```python
from build123d import *

# Parameters (mm, degrees)
BOSS_EXTRUDE1_DEPTH = 17.78
SKETCH4_R           = 1.905
SKETCH4_R_2         = 1.1
SKETCH4_W           = 3.81
SKETCH4_H           = 6.35
CUT_EXTRUDE1_DEPTH  = 7.62
BOSS_EXTRUDE2_DEPTH = 1.27
BOSS_EXTRUDE3_DEPTH = 1.27
FILLET1_R           = 3.81


with BuildPart() as part:
    # Sketch3 → Boss-Extrude1 (new body)
    with BuildSketch(Plane(origin=(0, 0, 0), x_dir=(1, 0, 0), z_dir=(0, 1, 0))):
        Polygon((0, 20.32), (57.15, 7.62), (57.15, -7.62), (0, -20.32), (0, -17.718039675), (54.61, -5.58248412), (54.61, 5.58248412), (0, 17.718039675), align=None)
    extrude(amount=BOSS_EXTRUDE1_DEPTH)

    # Sketch4 → Cut-Extrude1 (cut)
    with BuildSketch(Plane(origin=(57.15, 0, 0), x_dir=(0, 0, -1), z_dir=(1, 0, 0))):
        with Locations((0, 8.89)):
            Circle(SKETCH4_R)
        with Locations((-3.181980515, 12.071980515)):
            Circle(SKETCH4_R_2)
        with Locations((3.181980515, 12.071980515)):
            Circle(SKETCH4_R_2)
        with Locations((3.181980515, 5.708019485)):
            Circle(SKETCH4_R_2)
        with Locations((-3.181980515, 5.708019485)):
            Circle(SKETCH4_R_2)
        with Locations((7.62, 8.89)):
            Rectangle(SKETCH4_W, SKETCH4_H)
    extrude(amount=-CUT_EXTRUDE1_DEPTH, mode=Mode.SUBTRACT)

    # Sketch5 → Boss-Extrude2 (add)
    with BuildSketch(Plane(origin=(0, 17.78, 0), x_dir=(1, 0, 0), z_dir=(0, 1, 0))):
        Polygon((0, 20.32), (0, -20.32), (57.15, -7.62), (57.15, 7.62), align=None)
    extrude(amount=BOSS_EXTRUDE2_DEPTH)

    # Sketch6 → Boss-Extrude3 (add)
    with BuildSketch(Plane.XZ):
        Polygon((0, 20.32), (0, -20.32), (57.15, -7.62), (57.15, 7.62), align=None)
    extrude(amount=BOSS_EXTRUDE3_DEPTH)

    # Fillet1
    fillet1_edges = [part.edges().sort_by_distance(p)[0] for p in [
        (28.575, 19.05, -13.97),
        (28.575, 19.05, 13.97),
        (28.575, -1.27, 13.97),
        (28.575, -1.27, -13.97),
    ]]
    fillet(fillet1_edges, radius=FILLET1_R)


solid = part.part
```
Source: CAD feature listing. Evaluate the final solid. Frame: model axes, mm. A direction names the side the tool comes from. Coordinates: 2 decimals unless noted, no trailing zeros. Write each loop counter-clockwise with the first axis right and the second up, starting at its lowest first coordinate (ties: lowest second). Pieces come first, ordered by that corner, then holes. Notation, with made-up numbers: (-26.5, -21.75) -> (-19.5, -21.75) arc R14 cw to (-19.5, -9.75) -> close; hole circle Ø8 at (25, 26.25). An arc over 180 degrees is marked (long way). Return JSON: item names as keys, results as strings. Group by question number.
1) Contact query for flat-ended pins moving along their axis: P1, Ø2, axis at y = 10.5, z = -8.5, coming from the +X side; P2, Ø1.3, axis at y = 5.71, z = -3.18, coming from the -X side; P3, Ø5, axis at y = 8.89, z = 0, coming from the -X side; P4, Ø3, axis at x = 52.5, z = -8, coming from the +Y side. Output: stop coordinate, or through.
2) Ray query, line 1 along Y through (x, z) = (26.5, -6); line 2 along X through (y, z) = (10.25, -2); line 3 along Z through (x, y) = (29.5, 0.5). Return the intervals inside material, ascending.
3) Section query B-B, the plane y = 8.89. Return loops of the section in (x, z) (3 decimals).
4) Set-up query: faces 1 (the face through (49.53, 9, -8)), 2 (the face through (56, 9, -5.715)), 3 (the face through (28.17, 8.98, -14.06)), 4 (the face through (21, 0, 0)), 5 (the face through (55.9, 10.78, 0.25)). Return all of +Z, -Z, +X, -X, +Y, -Y with unobstructed straight access to the full face (end or side cutting, diameter ignored); none if empty.
5) Section query A-A, the plane z = 0. Return loops of the section in (x, y) (3 decimals), plus the area to 3 significant figures.
From the geometry:
{
 "1": {"P1": "x = 49.53", "P2": "through", "P3": "x = 54.61", "P4": "y = 18.66"},
 "2": {"line 1": "-1.27 to 0, 17.78 to 19.05", "line 2": "54.61 to 57.15", "line 3": "-13.16 to -11.16, 11.16 to 13.16"},
 "3": {"outline": "(0, -20.32) -> (49.53, -9.313) -> (49.53, -6.711) -> (0, -17.718) -> close; (0, 17.718) -> (54.61, 5.582) -> (54.61, 1.905) -> (57.15, 1.905) -> (57.15, 7.62) -> (0, 20.32) -> close; (54.014, -5.715) -> (57.15, -5.715) -> (57.15, -1.905) -> (54.61, -1.905) -> (54.61, -5.582) -> close"},
 "4": {"face 1": "-Z, +X", "face 2": "-Z, +X, -X", "face 3": "-Z, +X, +Y, -Y", "face 4": "-X", "face 5": "+X, -X"},
 "5": {"outline": "(0, -1.27) -> (57.15, -1.27) -> (57.15, 6.985) -> (54.61, 6.985) -> (54.61, 0) -> (0, 0) -> close; (0, 17.78) -> (54.61, 17.78) -> (54.61, 10.795) -> (57.15, 10.795) -> (57.15, 19.05) -> (0, 19.05) -> close", "area": "181 mm²"}
}
